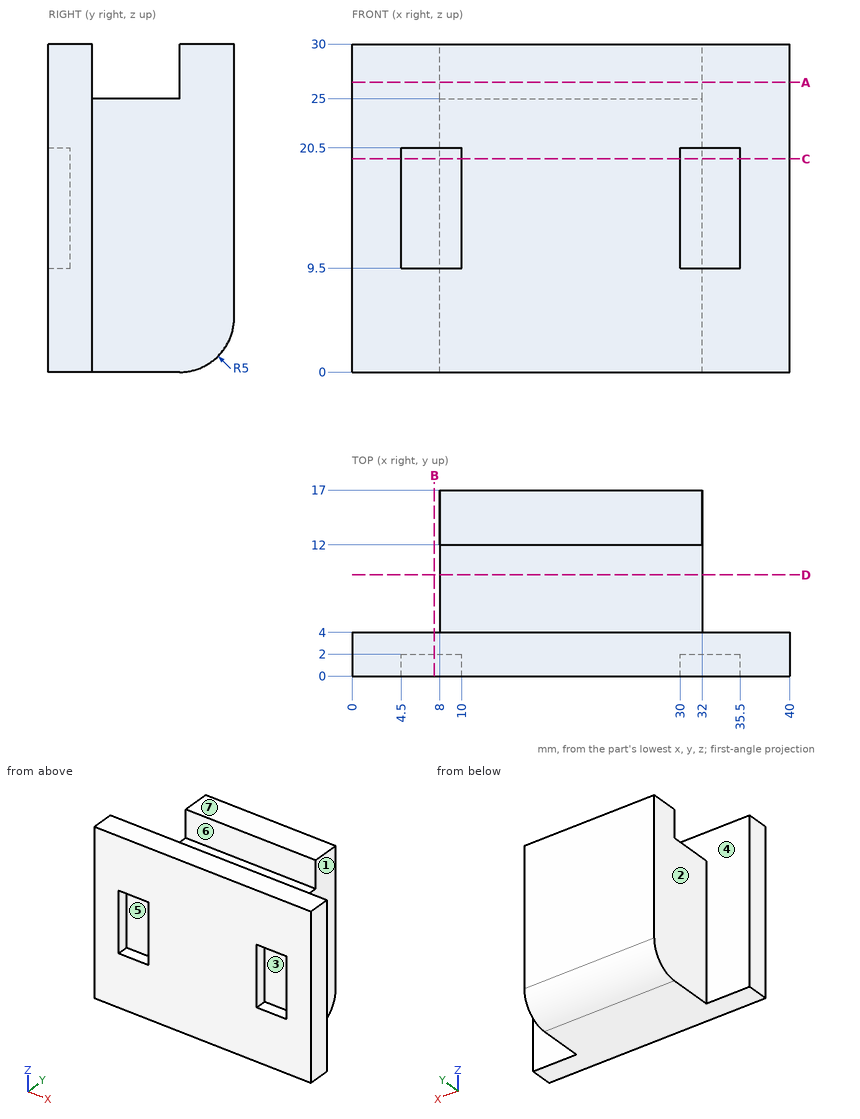
Part print with two shaded views. Sizes in mm from the minimum x, y, z corner. A direction names the side the tool comes from. Coordinates: 2 decimals unless noted, no trailing zeros. Order: outer loops, then holes, each group sorted by start corner. A loop starts at its lowest first (then second) coordinate and runs counter-clockwise, first axis right, second up.
(1) Saw through at C-C, the plane z = 19.5. Write the cut outline in (x, y).
Solution:
outline: (0, 0) - (4.5, 0) - (4.5, 2) - (10, 2) - (10, 0) - (30, 0) - (30, 2) - (35.5, 2) - (35.5, 0) - (40, 0) - (40, 4) - (32, 4) - (32, 17) - (8, 17) - (8, 4) - (0, 4) - close
(2) Which spindle directions (+Z, -Z, +X, -X, +Y, -Y) get a long thin tool onto all of the face, cutting with end or side? Do the marked faces 1, 2, 3 and 4. Say none if no direction does.
Solution:
face 1: +Z, -Z, +X, +Y
face 2: +Z, -Z, -X, +Y
face 3: -Y
face 4: +Z
(3) Mould opens along Y. For the marked faces 5, 6 and 7 say: released by +Y, released by -Y, zero draft, split by the parting line, or undercut.
Solution:
face 5: released by -Y
face 6: undercut
face 7: zero draft
(4) Saw through at B-B, the plane x = 7.5. Write the cut outline in (y, z).
Solution:
outline: (0, 0) - (4, 0) - (4, 30) - (0, 30) - (0, 20.5) - (2, 20.5) - (2, 9.5) - (0, 9.5) - close
(5) Saw through at A-A, the plane z = 26.5. Write the cut outline in (x, y).
Solution:
outline: (0, 0) - (40, 0) - (40, 4) - (0, 4) - close; (8, 12) - (32, 12) - (32, 17) - (8, 17) - close
(6) Pin check, flat tips, straight feed: pin 1 Ø1.5 at (y, z) = (14, 26.5) entering from +X; pin 2 Ø4 at (y, z) = (13, 21) entering from -X. Stop position of each tip, or through.
Solution:
pin 1: stops at x = 32
pin 2: stops at x = 8
(7) Drill centre lines: L1, parallel to Y at x = 15, z = 28.25; L2, parallel to Z at x = 24.5, y = 9.25; L3, parallel to Y at x = 8.5, z = 16.75. Where is each one in solid material? Low to high.
Solution:
L1: y = 0 to 4, 12 to 17
L2: z = 0 to 25
L3: y = 2 to 17
(8) Saw through at D-D, the plane y = 9.25. Write the cut outline in (x, z), and give its area (3 significant figures).
Solution:
outline: (8, 0) - (32, 0) - (32, 25) - (8, 25) - close
area: 600 mm2
